Could you check a few things on this model? Use its own coordinates, in mm. Coordinates: 2 decimals unless noted, no trailing zeros. Order: outer loops, then holes, each group sorted by start corner. A loop starts at its lowest first (then second) coordinate and runs counter-clockwise, first axis right, second up. Notation, with made-up numbers: (37.5, 26.5) -> (62.5, 26.5) arc R14 cw to (62.5, 36.5) -> close; hole circle Ø6 at (63, 67.5). An arc over 180 degrees is marked (long way). Use a Markdown table: item, result. Add a question column.
1) Will these pins go through, and if not, where does the flat tip stop? pin 1 Ø2 at (x, z) = (-347.5, 2.5) entering from +Y; pin 2 Ø1.4 at (y, z) = (0, 3) entering from -X; pin 3 Ø1.4 at (y, z) = (-0.5, 3) entering from +X.
2) If I drill on L1, parallel to Y at x = -296, z = 2.75; L2, parallel to Y at x = -313, z = 0.5; L3, parallel to X at y = -17, z = 3.5, over which ranges is the centre line in solid material (lowest first)? Write a range as [from, to].
3) If we section it at B-B (y = -182): Write out the boundary of the cut face in (x, z), plus the area to 3 significant figures.
4) If we section it at C-C (z = 5.25): Write out the boundary of the cut face in (x, y), plus the area to 3 significant figures.
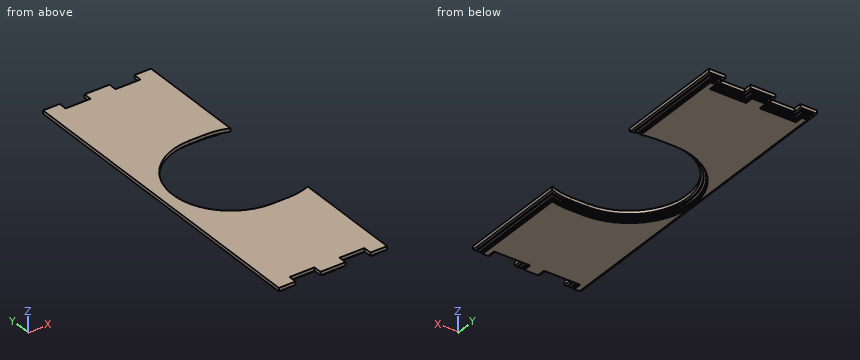
```python
from build123d import *

# Parameters (mm, degrees)
SKETCH1_W           = 82.55
SKETCH1_H           = 251.46
BOSS_EXTRUDE1_DEPTH = 6.35
SKETCH2_W           = 19.05
SKETCH2_H           = 6.35
CUT_EXTRUDE2_DEPTH  = 6.35
SKETCH5_W           = 19.05
SKETCH5_H           = 6.35
CUT_EXTRUDE4_DEPTH  = 6.35
CUT_EXTRUDE5_DEPTH  = 7.35
CUT_EXTRUDE6_DEPTH  = 3.81
CUT_EXTRUDE7_DEPTH  = 2.54
CUT_EXTRUDE8_DEPTH  = 1.27


with BuildPart() as part:
    # Sketch1 → Boss-Extrude1 (new body)
    with BuildSketch(Plane.XY):
        with Locations((-333.375, -120.65)):
            Rectangle(SKETCH1_W, SKETCH1_H)
    extrude(amount=BOSS_EXTRUDE1_DEPTH)

    # Sketch2 → Cut-Extrude2 (cut)
    with BuildSketch(Plane(origin=(0, 5.08, 0), x_dir=(1, 0, 0), z_dir=(0, 1, 0))):
        with Locations((-352.425, -3.175)):
            Rectangle(SKETCH2_W, SKETCH2_H)
        with Locations((-314.325, -3.175)):
            Rectangle(SKETCH2_W, SKETCH2_H)
    extrude(amount=-CUT_EXTRUDE2_DEPTH, mode=Mode.SUBTRACT)

    # Sketch5 → Cut-Extrude4 (cut)
    with BuildSketch(Plane.XZ.offset(246.38)):
        with Locations((-352.425, 3.175)):
            Rectangle(SKETCH5_W, SKETCH5_H)
        with Locations((-314.325, 3.175)):
            Rectangle(SKETCH5_W, SKETCH5_H)
    extrude(amount=-CUT_EXTRUDE4_DEPTH, mode=Mode.SUBTRACT)

    # Sketch6 → Cut-Extrude5 (cut, through all)
    with BuildSketch(Plane.XY.offset(6.35)):
        with BuildLine():
            Line((-321.31, -165.1), (-308.61, -165.1))
            ThreePointArc((-308.61, -165.1), (-264.16, -120.65), (-308.61, -76.2))
            Line((-308.61, -76.2), (-321.31, -76.2))
            ThreePointArc((-321.31, -76.2), (-365.76, -120.65), (-321.31, -165.1))
        make_face()
    extrude(amount=-CUT_EXTRUDE5_DEPTH, mode=Mode.SUBTRACT)

    # Sketch8 → Cut-Extrude6 (cut)
    with BuildSketch(Plane(origin=(0, 0, 0), x_dir=(-1, 0, 0), z_dir=(0, 0, -1))):
        with BuildLine():
            Line((374.65, 5.08), (361.95, 5.08))
            Line((361.95, 5.08), (361.95, -1.27))
            Line((361.95, -1.27), (342.9, -1.27))
            Line((342.9, -1.27), (342.9, 5.08))
            Line((342.9, 5.08), (323.85, 5.08))
            Line((323.85, 5.08), (323.85, -1.27))
            Line((323.85, -1.27), (304.8, -1.27))
            Line((304.8, -1.27), (304.8, 5.08))
            Line((304.8, 5.08), (292.1, 5.08))
            Line((292.1, 5.08), (292.1, -79.379884904))
            ThreePointArc((292.1, -79.379884904), (300.20327995, -77.002210159), (308.61, -76.2))
            Line((308.61, -76.2), (321.31, -76.2))
            ThreePointArc((321.31, -76.2), (365.76, -120.65), (321.31, -165.1))
            Line((321.31, -165.1), (308.61, -165.1))
            ThreePointArc((308.61, -165.1), (300.20327995, -164.297789841), (292.1, -161.920115096))
            Line((292.1, -161.920115096), (292.1, -246.38))
            Line((292.1, -246.38), (304.8, -246.38))
            Line((304.8, -246.38), (304.8, -240.03))
            Line((304.8, -240.03), (323.85, -240.03))
            Line((323.85, -240.03), (323.85, -246.38))
            Line((323.85, -246.38), (342.9, -246.38))
            Line((342.9, -246.38), (342.9, -240.03))
            Line((342.9, -240.03), (361.95, -240.03))
            Line((361.95, -240.03), (361.95, -246.38))
            Line((361.95, -246.38), (374.65, -246.38))
            Line((374.65, -246.38), (374.65, 5.08))
        make_face()
        with BuildLine():
            Line((321.31, -74.422), (308.61, -74.422))
            ThreePointArc((308.61, -74.422), (301.146068779, -75.02853888), (293.878, -76.832239217))
            Line((293.878, -76.832239217), (293.878, 3.302))
            Line((293.878, 3.302), (303.022, 3.302))
            Line((303.022, 3.302), (303.022, -3.048))
            Line((303.022, -3.048), (325.628, -3.048))
            Line((325.628, -3.048), (325.628, 3.302))
            Line((325.628, 3.302), (341.122, 3.302))
            Line((341.122, 3.302), (341.122, -3.048))
            Line((341.122, -3.048), (363.728, -3.048))
            Line((363.728, -3.048), (363.728, 3.302))
            Line((363.728, 3.302), (372.872, 3.302))
            Line((372.872, 3.302), (372.872, -244.602))
            Line((372.872, -244.602), (363.728, -244.602))
            Line((363.728, -244.602), (363.728, -238.252))
            Line((363.728, -238.252), (341.122, -238.252))
            Line((341.122, -238.252), (341.122, -244.602))
            Line((341.122, -244.602), (325.628, -244.602))
            Line((325.628, -244.602), (325.628, -238.252))
            Line((325.628, -238.252), (303.022, -238.252))
            Line((303.022, -238.252), (303.022, -244.602))
            Line((303.022, -244.602), (293.878, -244.602))
            Line((293.878, -244.602), (293.878, -164.467760783))
            ThreePointArc((293.878, -164.467760783), (301.146068779, -166.27146112), (308.61, -166.878))
            Line((308.61, -166.878), (321.31, -166.878))
            ThreePointArc((321.31, -166.878), (367.538, -120.65), (321.31, -74.422))
        make_face(mode=Mode.SUBTRACT)
    extrude(amount=-CUT_EXTRUDE6_DEPTH, mode=Mode.SUBTRACT)

    # Sketch9 → Cut-Extrude7 (cut)
    with BuildSketch(Plane(origin=(0, 0, 0), x_dir=(-1, 0, 0), z_dir=(0, 0, -1))):
        with BuildLine():
            Line((308.61, -74.422), (321.31, -74.422))
            ThreePointArc((321.31, -74.422), (367.538, -120.65), (321.31, -166.878))
            Line((321.31, -166.878), (308.61, -166.878))
            ThreePointArc((308.61, -166.878), (301.146068779, -166.27146112), (293.878, -164.467760783))
            Line((293.878, -164.467760783), (293.878, -244.602))
            Line((293.878, -244.602), (303.022, -244.602))
            Line((303.022, -244.602), (303.022, -238.252))
            Line((303.022, -238.252), (325.628, -238.252))
            Line((325.628, -238.252), (325.628, -244.602))
            Line((325.628, -244.602), (341.122, -244.602))
            Line((341.122, -244.602), (341.122, -238.252))
            Line((341.122, -238.252), (363.728, -238.252))
            Line((363.728, -238.252), (363.728, -244.602))
            Line((363.728, -244.602), (372.872, -244.602))
            Line((372.872, -244.602), (372.872, 3.302))
            Line((372.872, 3.302), (363.728, 3.302))
            Line((363.728, 3.302), (363.728, -3.048))
            Line((363.728, -3.048), (341.122, -3.048))
            Line((341.122, -3.048), (341.122, 3.302))
            Line((341.122, 3.302), (325.628, 3.302))
            Line((325.628, 3.302), (325.628, -3.048))
            Line((325.628, -3.048), (303.022, -3.048))
            Line((303.022, -3.048), (303.022, 3.302))
            Line((303.022, 3.302), (293.878, 3.302))
            Line((293.878, 3.302), (293.878, -76.832239217))
            ThreePointArc((293.878, -76.832239217), (301.146068779, -75.02853888), (308.61, -74.422))
        make_face()
        with BuildLine():
            Line((295.656, -242.824), (295.656, -166.875208707))
            ThreePointArc((295.656, -166.875208707), (302.072084934, -168.208718471), (308.61, -168.656))
            Line((308.61, -168.656), (321.31, -168.656))
            ThreePointArc((321.31, -168.656), (369.316, -120.65), (321.31, -72.644))
            Line((321.31, -72.644), (308.61, -72.644))
            ThreePointArc((308.61, -72.644), (302.072084934, -73.091281529), (295.656, -74.424791293))
            Line((295.656, -74.424791293), (295.656, 1.524))
            Line((295.656, 1.524), (301.244, 1.524))
            Line((301.244, 1.524), (301.244, -4.826))
            Line((301.244, -4.826), (327.406, -4.826))
            Line((327.406, -4.826), (327.406, 1.524))
            Line((327.406, 1.524), (339.344, 1.524))
            Line((339.344, 1.524), (339.344, -4.826))
            Line((339.344, -4.826), (365.506, -4.826))
            Line((365.506, -4.826), (365.506, 1.524))
            Line((365.506, 1.524), (371.094, 1.524))
            Line((371.094, 1.524), (371.094, -242.824))
            Line((371.094, -242.824), (365.506, -242.824))
            Line((365.506, -242.824), (365.506, -236.474))
            Line((365.506, -236.474), (339.344, -236.474))
            Line((339.344, -236.474), (339.344, -242.824))
            Line((339.344, -242.824), (327.406, -242.824))
            Line((327.406, -242.824), (327.406, -236.474))
            Line((327.406, -236.474), (301.244, -236.474))
            Line((301.244, -236.474), (301.244, -242.824))
            Line((301.244, -242.824), (295.656, -242.824))
        make_face(mode=Mode.SUBTRACT)
    extrude(amount=-CUT_EXTRUDE7_DEPTH, mode=Mode.SUBTRACT)

    # Sketch10 → Cut-Extrude8 (cut)
    with BuildSketch(Plane(origin=(0, 0, 0), x_dir=(-1, 0, 0), z_dir=(0, 0, -1))):
        with BuildLine():
            Line((295.656, -166.875208707), (295.656, -242.824))
            Line((295.656, -242.824), (301.244, -242.824))
            Line((301.244, -242.824), (301.244, -236.474))
            Line((301.244, -236.474), (327.406, -236.474))
            Line((327.406, -236.474), (327.406, -242.824))
            Line((327.406, -242.824), (339.344, -242.824))
            Line((339.344, -242.824), (339.344, -236.474))
            Line((339.344, -236.474), (365.506, -236.474))
            Line((365.506, -236.474), (365.506, -242.824))
            Line((365.506, -242.824), (371.094, -242.824))
            Line((371.094, -242.824), (371.094, 1.524))
            Line((371.094, 1.524), (365.506, 1.524))
            Line((365.506, 1.524), (365.506, -4.826))
            Line((365.506, -4.826), (339.344, -4.826))
            Line((339.344, -4.826), (339.344, 1.524))
            Line((339.344, 1.524), (327.406, 1.524))
            Line((327.406, 1.524), (327.406, -4.826))
            Line((327.406, -4.826), (301.244, -4.826))
            Line((301.244, -4.826), (301.244, 1.524))
            Line((301.244, 1.524), (295.656, 1.524))
            Line((295.656, 1.524), (295.656, -74.424791293))
            ThreePointArc((295.656, -74.424791293), (302.072084934, -73.091281529), (308.61, -72.644))
            Line((308.61, -72.644), (321.31, -72.644))
            ThreePointArc((321.31, -72.644), (369.316, -120.65), (321.31, -168.656))
            Line((321.31, -168.656), (308.61, -168.656))
            ThreePointArc((308.61, -168.656), (302.072084934, -168.208718471), (295.656, -166.875208707))
        make_face()
        with BuildLine():
            Line((308.61, -169.418), (321.31, -169.418))
            ThreePointArc((321.31, -169.418), (370.078, -120.65), (321.31, -71.882))
            Line((321.31, -71.882), (308.61, -71.882))
            ThreePointArc((308.61, -71.882), (302.465022664, -72.270695772), (296.418, -73.430587043))
            Line((296.418, -73.430587043), (296.418, 0.762))
            Line((296.418, 0.762), (300.482, 0.762))
            Line((300.482, 0.762), (300.482, -5.588))
            Line((300.482, -5.588), (328.168, -5.588))
            Line((328.168, -5.588), (328.168, 0.762))
            Line((328.168, 0.762), (338.582, 0.762))
            Line((338.582, 0.762), (338.582, -5.588))
            Line((338.582, -5.588), (366.268, -5.588))
            Line((366.268, -5.588), (366.268, 0.762))
            Line((366.268, 0.762), (370.332, 0.762))
            Line((370.332, 0.762), (370.332, -242.062))
            Line((370.332, -242.062), (366.268, -242.062))
            Line((366.268, -242.062), (366.268, -235.712))
            Line((366.268, -235.712), (338.582, -235.712))
            Line((338.582, -235.712), (338.582, -242.062))
            Line((338.582, -242.062), (328.168, -242.062))
            Line((328.168, -242.062), (328.168, -235.712))
            Line((328.168, -235.712), (300.482, -235.712))
            Line((300.482, -235.712), (300.482, -242.062))
            Line((300.482, -242.062), (296.418, -242.062))
            Line((296.418, -242.062), (296.418, -167.869412957))
            ThreePointArc((296.418, -167.869412957), (302.465022664, -169.029304228), (308.61, -169.418))
        make_face(mode=Mode.SUBTRACT)
    extrude(amount=-CUT_EXTRUDE8_DEPTH, mode=Mode.SUBTRACT)


solid = part.part
```
Answer sheet:
| question | item | result |
|---|---|---|
| 1 | pin 1 | y = -3.05 |
| 1 | pin 2 | x = -372.87 |
| 1 | pin 3 | x = -293.88 |
| 2 | L1 | [-244.6, -165.12], [-76.18, 3.3] |
| 2 | L2 | [-235.71, -169.42], [-71.88, -5.59] |
| 2 | L3 | [-372.87, -293.88] |
| 3 | outline | (-374.65, 3.81) -> (-372.87, 3.81) -> (-372.87, 2.54) -> (-371.09, 2.54) -> (-371.09, 1.27) -> (-370.33, 1.27) -> (-370.33, 0) -> (-296.42, 0) -> (-296.42, 1.27) -> (-295.66, 1.27) -> (-295.66, 2.54) -> (-293.88, 2.54) -> (-293.88, 3.81) -> (-292.1, 3.81) -> (-292.1, 6.35) -> (-374.65, 6.35) -> close |
| 3 | area | 500 mm2 |
| 4 | outline | (-374.65, -246.38) -> (-361.95, -246.38) -> (-361.95, -240.03) -> (-342.9, -240.03) -> (-342.9, -246.38) -> (-323.85, -246.38) -> (-323.85, -240.03) -> (-304.8, -240.03) -> (-304.8, -246.38) -> (-292.1, -246.38) -> (-292.1, -161.92) arc R44.45 cw to (-308.61, -165.1) -> (-321.31, -165.1) arc R44.45 cw to (-321.31, -76.2) -> (-308.61, -76.2) arc R44.45 cw to (-292.1, -79.38) -> (-292.1, 5.08) -> (-304.8, 5.08) -> (-304.8, -1.27) -> (-323.85, -1.27) -> (-323.85, 5.08) -> (-342.9, 5.08) -> (-342.9, -1.27) -> (-361.95, -1.27) -> (-361.95, 5.08) -> (-374.65, 5.08) -> close |
| 4 | area | 14,600 mm2 |
